from build123d import *

# Parameters (mm, degrees)
SKETCH1_R           = 42.5
SKETCH1_R_2         = 32
SKETCH1_R_3         = 1.5
BOSS_EXTRUDE1_DEPTH = 4
SKETCH2_R           = 2.05
SKETCH2_R_2         = 7
BOSS_EXTRUDE2_DEPTH = 4


with BuildPart() as part:
    # Sketch1 → Boss-Extrude1 (new body)
    with BuildSketch(Plane.XY):
        Circle(SKETCH1_R)
        Circle(SKETCH1_R_2, mode=Mode.SUBTRACT)
        with Locations((0, 37.066662977)):
            Circle(SKETCH1_R_3, mode=Mode.SUBTRACT)
        with Locations((35.252491362, 11.454228785)):
            Circle(SKETCH1_R_3, mode=Mode.SUBTRACT)
        with Locations((21.78723785, -29.987560273)):
            Circle(SKETCH1_R_3, mode=Mode.SUBTRACT)
        with Locations((-21.78723785, -29.987560273)):
            Circle(SKETCH1_R_3, mode=Mode.SUBTRACT)
        with Locations((-35.252491362, 11.454228785)):
            Circle(SKETCH1_R_3, mode=Mode.SUBTRACT)
    extrude(amount=BOSS_EXTRUDE1_DEPTH)

    # Sketch2 → Boss-Extrude2 (add, through all)
    with BuildSketch(Plane.XY.offset(4)):
        with BuildLine():
            Line((-9.16515139, 4), (-31.749015733, 4))
            ThreePointArc((-31.749015733, 4), (-32, 0), (-31.749015733, -4))
            Line((-31.749015733, -4), (-9.16515139, -4))
            ThreePointArc((-9.16515139, -4), (-7.071067812, -7.071067812), (-4, -9.16515139))
            Line((-4, -9.16515139), (-4, -31.749015733))
            ThreePointArc((-4, -31.749015733), (0, -32), (4, -31.749015733))
            Line((4, -31.749015733), (4, -9.16515139))
            ThreePointArc((4, -9.16515139), (7.071067812, -7.071067812), (9.16515139, -4))
            Line((9.16515139, -4), (31.749015733, -4))
            ThreePointArc((31.749015733, -4), (32, 0), (31.749015733, 4))
            Line((31.749015733, 4), (9.16515139, 4))
            ThreePointArc((9.16515139, 4), (7.071067812, 7.071067812), (4, 9.16515139))
            Line((4, 9.16515139), (4, 31.749015733))
            ThreePointArc((4, 31.749015733), (0, 32), (-4, 31.749015733))
            Line((-4, 31.749015733), (-4, 9.16515139))
            ThreePointArc((-4, 9.16515139), (-7.071067812, 7.071067812), (-9.16515139, 4))
        make_face()
        with Locations((0, 22)):
            Circle(SKETCH2_R, mode=Mode.SUBTRACT)
        with Locations((22, 0)):
            Circle(SKETCH2_R, mode=Mode.SUBTRACT)
        with Locations((0, -22)):
            Circle(SKETCH2_R, mode=Mode.SUBTRACT)
        with Locations((-22, 0)):
            Circle(SKETCH2_R, mode=Mode.SUBTRACT)
        Circle(SKETCH2_R_2, mode=Mode.SUBTRACT)
    extrude(amount=-BOSS_EXTRUDE2_DEPTH)


solid = part.part
Geometry: final body of the model. Coordinates: model frame, mm. Give positions to 0.01 mm unless a question says otherwise; leave off trailing zeros. Write each loop counter-clockwise with the first axis right and the second up, starting at its lowest first coordinate (ties: lowest second). Pieces come first, ordered by that corner, then holes.
(1) Cut plane A-A, the plane x = 0. Return loops of the section in (y, z), then the cut area to 3 significant figures.
(2) Ray query, line 1 (Y direction, x = 0, z = 2.45); line 2 (X direction, y = -14.5, z = 0.4); line 3 (Y direction, x = 5.5, z = 2.1). Return the intervals inside material, ascending.
(3) Cut plane B-B, the plane y = 0. Return loops of the section in (x, z), then the cut area to 3 significant figures.
(4) Cut plane D-D, the plane z = 2.25. Give the number of separate pieces and of enclosed holes in the cut face, then the cut area to 3 significant figures.
(5) Cut plane C-C, the plane y = -18. Return loops of the section in (x, z), then the cut area to 3 significant figures.
(6) First-contact query: P1, Ø1.2, axis at x = -18.5, z = 2.5, coming from the -Y side; P2, Ø2.5, axis at x = 35.25, y = 11.45, coming from the -Z side; P3, Ø1, axis at x = -19.5, z = 2.5, coming from the +Y side. Flat tips, straight axial feed; report the tip coordinate or a pass-through.
(7) Mould query, pull axis X, two halves, no side actions, for faces 1 (the cylindrical face through (-1.5, -20.6, 2)), 2 (the flat face through (-1, -9, 0)), 3 (the cylindrical face through (-20.357, -29.537, 1.972)), 4 (the cylindrical face through (-33.727, -25.861, 1.972)). Classes: released by +X, released by -X, zero draft, split by the parting line, or undercut.
Values follow:
1. outline: (-42.5, 0) - (-24.05, 0) - (-24.05, 4) - (-42.5, 4) - close; (-19.95, 0) - (-7, 0) - (-7, 4) - (-19.95, 4) - close; (7, 0) - (19.95, 0) - (19.95, 4) - (7, 4) - close; (24.05, 0) - (35.57, 0) - (35.57, 4) - (24.05, 4) - close; (38.57, 0) - (42.5, 0) - (42.5, 4) - (38.57, 4) - close
1. area: 239 mm2
2. line 1: y = -42.5 to -24.05, -19.95 to -7, 7 to 19.95, 24.05 to 35.57, 38.57 to 42.5
2. line 2: x = -39.95 to -28.53, -4 to 4, 28.53 to 39.95
2. line 3: y = -42.14 to -31.52, -8.35 to -4.33, 4.33 to 8.35, 31.52 to 42.14
3. outline: (-42.5, 0) - (-24.05, 0) - (-24.05, 4) - (-42.5, 4) - close; (-19.95, 0) - (-7, 0) - (-7, 4) - (-19.95, 4) - close; (7, 0) - (19.95, 0) - (19.95, 4) - (7, 4) - close; (24.05, 0) - (42.5, 0) - (42.5, 4) - (24.05, 4) - close
3. area: 251 mm2
4. separate pieces: 1
4. enclosed holes: 14
4. area: 3,240 mm2
5. outline: (-38.5, 0) - (-26.46, 0) - (-26.46, 4) - (-38.5, 4) - close; (-4, 0) - (4, 0) - (4, 4) - (-4, 4) - close; (26.46, 0) - (38.5, 0) - (38.5, 4) - (26.46, 4) - close
5. area: 128 mm2
6. P1: stops at y = -38.55
6. P2: passes through
6. P3: stops at y = 38.02
7. face 1: undercut
7. face 2: zero draft
7. face 3: undercut
7. face 4: split by the parting line
